The model under review builds one solid part; all positions refer to its coordinate system, in mm. A direction names the side the tool comes from. Round coordinates to 2 decimals unless told otherwise and drop trailing zeros. Loops run counter-clockwise (first coordinate to the right, second up) from the corner with the lowest first, then second, coordinate; pieces in that order, holes last. Notation, with made-up numbers: M -31,69 L -27,69 A23 ccw -27,81 Z; hole C 18.5,36 d5. An arc over 180 degrees is marked long. Answer as a JSON object with one key per item and string values. Group by question number.
Item 1: Consider section A-A (x = -27.5). Give the boundary of the cut face in (y, z).
Item 2: The part is to be moulded in two halves that separate along Z. For faces 1 (the face through (-12.156, -8.092, 28.801)), 2 (the face through (-19, 151, 65.188)), 3 (the face through (-1, 8, 0)), say which applies: +Z half, -Z half, draft (parallel to the pull), parting line (faces both ways), or undercut.
Item 3: Tool access review of faces 4 (the face through (32, 0, 29)), 5 (the face through (-32, 0, 29)), 6 (the face through (-14.732, -27, 29)), 7 (the face through (-19, 112, 0)): name each direction out of +Z, -Z, +X, -X, +Y, -Y from which nothing blocks a thin tool from reaching the whole face with its end or side.
Item 4: Consider section C-C (x = 23). Give the boundary of the cut face in (y, z).
Item 5: To check wall thickness, follow line 1 (Y direction, x = -6.5, z = 2.5); line 2 (Y direction, x = 29, z = 46.5); line 3 (Z direction, x = -12, y = 127). State the ranges of each line that lie inside material, in increasing order.
Item 6: Consider section B-B (y = -30). Give the boundary of the cut face in (x, z).
Item 7: Consider section D-D (z = 28.5). Give the boundary of the cut face in (x, y).
Item 8: Insertion check: P1, Ø18, axis at y = 124, z = 32.5, coming from the -X side; P2, Ø4, axis at x = -2, y = 85, coming from the -Z side; P3, Ø3, axis at x = 2.5, y = 22, coming from the +Z side. Each pin has a flat end and moves straight along its axis. Give the tip position at first contact, or say it passes through.
```python
from build123d import *

# Parameters (mm, degrees)
F1_DEPTH = 58.42
F3_DEPTH = 31.242
F4_W     = 12.51252
F4_H     = 17.674709
F5_DEPTH = 25.4
F6_SIZE  = 5.08


with BuildPart() as f1:
    # F0 (on Top) → F1 (new body)
    with BuildSketch(Plane.XY):
        Polygon((-43.942, 0), (-43.942, -43.688), (-14.732, -43.688), (-14.732, -5.588), (0, -5.588), (14.732, -5.588), (14.732, -43.688), (43.942, -43.688), (43.942, 0), (14.732, 0), (14.732, 87.884), (0, 87.884), (-14.732, 87.884), (-14.732, 0), align=None)
    extrude(amount=F1_DEPTH)

    # F2 (on Right) → F3 (join, symmetric)
    with BuildSketch(Plane.YZ):
        Polygon((87.884, 75.542652), (87.884, 58.42), (87.884, 54.577157), (87.884, 0), (87.884, -17.122652), (165.792628, -17.122652), (165.792628, 75.542652), align=None)
    extrude(amount=F3_DEPTH, both=True)

    # F4 (on face) → F5 (cut)
    with BuildSketch(Plane(origin=(-31.242, 0, 0), x_dir=(0, -1, 0), z_dir=(-1, 0, 0))):
        with Locations((-150.845341, 2.069356)):
            Rectangle(F4_W, F4_H)
        Polygon((-135.569647, 44.218883), (-135.569647, 29.21), (-135.569647, 14.201117), (-124.647684, 14.201117), (-124.647684, 0), (-99.536583, 0), (-99.536583, 21.531122), (-109.823912, 21.531122), (-109.823912, 29.21), (-109.823912, 36.888878), (-99.536583, 36.888878), (-99.536583, 58.42), (-124.647684, 58.42), (-124.647684, 44.218883), align=None)
        with Locations((-150.845341, 56.350644)):
            Rectangle(F4_W, F4_H)
    extrude(amount=-F5_DEPTH, mode=Mode.SUBTRACT)

    # F6
    f6_edges = [f1.edges().sort_by_distance(p)[0] for p in [
        (14.732, -5.588, 29.21),
        (-14.732, -5.588, 29.21),
        (-14.732, 0, 29.21),
        (14.732, 0, 29.21),
    ]]
    chamfer(f6_edges, length=F6_SIZE)


solid = f1.part
```
Geometry results:
{
 "1": {"outline": "M -43.69,0 L 0,0 L 0,58.42 L -43.69,58.42 Z; M 87.88,-17.12 L 165.79,-17.12 L 165.79,75.54 L 87.88,75.54 Z; hole M 99.54,0 L 124.65,0 L 124.65,14.2 L 135.57,14.2 L 135.57,44.22 L 124.65,44.22 L 124.65,58.42 L 99.54,58.42 L 99.54,36.89 L 109.82,36.89 L 109.82,21.53 L 99.54,21.53 Z; hole M 144.59,-6.77 L 157.1,-6.77 L 157.1,10.91 L 144.59,10.91 Z; hole M 144.59,47.51 L 157.1,47.51 L 157.1,65.19 L 144.59,65.19 Z"},
 "2": {"face 1": "draft", "face 2": "undercut", "face 3": "-Z half"},
 "3": {"face 4": "+Z, -Z, +X", "face 5": "+Z, -Z, -X", "face 6": "+Z, -Z, -Y", "face 7": "-X"},
 "4": {"outline": "M -43.69,0 L 0,0 L 0,58.42 L -43.69,58.42 Z; M 87.88,-17.12 L 165.79,-17.12 L 165.79,75.54 L 87.88,75.54 Z"},
 "5": {"line 1": "y = -5.59 to 99.54, 124.65 to 144.59, 157.1 to 165.79", "line 2": "y = -43.69 to 0, 87.88 to 165.79", "line 3": "z = -17.12 to 14.2, 44.22 to 75.54"},
 "6": {"outline": "M -43.94,0 L -14.73,0 L -14.73,58.42 L -43.94,58.42 Z; M 14.73,0 L 43.94,0 L 43.94,58.42 L 14.73,58.42 Z"},
 "7": {"outline": "M -43.94,-43.69 L -14.73,-43.69 L -14.73,-10.67 L -9.65,-5.59 L 9.65,-5.59 L 14.73,-10.67 L 14.73,-43.69 L 43.94,-43.69 L 43.94,0 L 19.81,0 L 14.73,5.08 L 14.73,87.88 L 31.24,87.88 L 31.24,165.79 L -31.24,165.79 L -31.24,135.57 L -5.84,135.57 L -5.84,109.82 L -31.24,109.82 L -31.24,87.88 L -14.73,87.88 L -14.73,5.08 L -19.81,0 L -43.94,0 Z"},
 "8": {"P1": "stops at x = -5.84", "P2": "stops at z = 0", "P3": "stops at z = 58.42"}
}
